The listing builds one solid part. Answer for the finished solid, in the listing's coordinates (mm). A direction names the side the tool comes from. Round coordinates to 2 decimals unless told otherwise and drop trailing zeros. Write each loop counter-clockwise with the first axis right and the second up, starting at its lowest first coordinate (ties: lowest second). Pieces come first, ordered by that corner, then holes. Notation, with made-up numbers: M 78,35 L 92,35 A17 ccw 92,67 Z; hole C -4,48.25 d4. An arc over 180 degrees is marked long. One line per item, written item: value. Start each with the question number.
(1) Consider probe 1 along Y at (x, z) = (-19, -5.5). Determine where the line is inside the solid, lowest interval first.
(2) Section B-B (z = 9.5) is taken. Determine the outline of the cut face in (x, y), plus the area to 3 significant figures.
(3) Section A-A (x = 0) is taken. Determine the outline of the cut face in (y, z).
(4) Section C-C (y = 15) is taken. Determine the outline of the cut face in (x, z), plus the area to 3 significant figures.
(5) Section D-D (x = -11) is taken. Determine the outline of the cut face in (y, z).
(6) For faces 1 (the cylindrical face through (-0.54, 17.26, -2.44)), 2 (the flat face through (-21, -17, 0)), determine the directions among +Z, -Z, +X, -X, +Y, -Y from which every point of the face is accessible in a straight line to the end or side of a thin tool.
(7) Given P1, Ø1.5, axis at x = 3, z = -3.5, coming from the +Y side; P2, Ø12.5, axis at x = -5.5, z = 4.5, coming from the +Y side, each flat-ended and moving along its own axis, determine where each tip first touches the part or whether it passes through.
```python
from build123d import *

# Parameters (mm, degrees)
F0_W     = 42
F0_H     = 42
F0_R     = 2.5
F1_DEPTH = 35
F2_DEPTH = 35


with BuildPart() as f1:
    # F0 (on Front) → F1 (new body)
    with BuildSketch(Plane.XZ):
        Rectangle(F0_W, F0_H)
        Circle(F0_R, mode=Mode.SUBTRACT)
        Circle(F0_R)
    extrude(amount=F1_DEPTH)

    # F0 (on Front) → F2 (join)
    with BuildSketch(Plane.XZ):
        Circle(F0_R)
    extrude(amount=-F2_DEPTH)


solid = f1.part
```
Recorded:
1. probe 1: y = -35 to 0
2. outline: M -21,-35 L 21,-35 L 21,0 L -21,0 Z
2. area: 1,470 mm2
3. outline: M -35,-21 L 0,-21 L 0,-2.5 L 35,-2.5 L 35,2.5 L 0,2.5 L 0,21 L -35,21 Z
4. outline: C 0,0 d5
4. area: 19.6 mm2
5. outline: M -35,-21 L 0,-21 L 0,21 L -35,21 Z
6. face 1: +Y
6. face 2: +Z, -Z, -X, +Y, -Y
7. P1: stops at y = 0
7. P2: stops at y = 35
